Work out the finished part from the listing and answer in its coordinate system (mm). A direction names the side the tool comes from. Coordinates: 2 decimals unless noted, no trailing zeros. Loops run counter-clockwise (first coordinate to the right, second up) from the corner with the lowest first, then second, coordinate; pieces in that order, holes last. Notation, with made-up numbers: M 48,62 L 95,62 A27 ccw 95,97 Z; hole C 29,52 d9. An arc over 180 degrees is marked long. Write each question's results on one line, items separated by ' | '.
```python
from build123d import *

# Parameters (mm, degrees)
BOSS_EXTRUDE1_DEPTH = 1.8
SKETCH3_R           = 1.6
CUT_EXTRUDE1_DEPTH  = 31.775680334
SKETCH4_R           = 2.65
BOSS_EXTRUDE2_DEPTH = 4
SKETCH5_R           = 1.65
CUT_EXTRUDE2_DEPTH  = 31.98229333
SKETCH7_R           = 4.5
SKETCH7_R_2         = 3.5
BOSS_EXTRUDE4_DEPTH = 2.2
CHAMFER2_SIZE       = 1


with BuildPart() as part:
    # Sketch1 → Boss-Extrude1 (new body)
    with BuildSketch(Plane(origin=(0, 0, 0), x_dir=(1, 0, 0), z_dir=(0, 1, 0))):
        Polygon((0, 0.2), (23.05, 0.2), (23.05, 4.2), (29.05, 4.2), (29.05, 10), (0, 10), (0, 4.2), align=None)
    extrude(amount=BOSS_EXTRUDE1_DEPTH)

    # Sketch3 → Cut-Extrude1 (cut, through all)
    with BuildSketch(Plane.XZ):
        with Locations(Location((3.5, -3.689750901, 0), (0, 0, 270))):
            Circle(SKETCH3_R)
    extrude(amount=-CUT_EXTRUDE1_DEPTH, mode=Mode.SUBTRACT)

    # Sketch4 → Boss-Extrude2 (add)
    with BuildSketch(Plane.XZ):
        with Locations(Location((15, -4.689750901, 0), (0, 0, 270))):
            Circle(SKETCH4_R)
    extrude(amount=-BOSS_EXTRUDE2_DEPTH)

    # Sketch5 → Cut-Extrude2 (cut, through all)
    with BuildSketch(Plane(origin=(0, 4, 0), x_dir=(1, 0, 0), z_dir=(0, 1, 0))):
        with Locations(Location((15, 4.689750901, 0), (0, 0, 270))):
            Circle(SKETCH5_R)
    extrude(amount=-CUT_EXTRUDE2_DEPTH, mode=Mode.SUBTRACT)

    # Sketch7 → Boss-Extrude4 (add)
    with BuildSketch(Plane(origin=(0, 1.8, 0), x_dir=(1, 0, 0), z_dir=(0, 1, 0))):
        with Locations(Location((15, 4.689750901, 0), (0, 0, 90))):
            Circle(SKETCH7_R)
        with Locations(Location((15, 4.689750901, 0), (0, 0, 90))):
            Circle(SKETCH7_R_2, mode=Mode.SUBTRACT)
    extrude(amount=BOSS_EXTRUDE4_DEPTH)

    # Chamfer2
    chamfer2_edges = [part.edges().sort_by_distance(p)[0] for p in [
        (23.05, 1.8, -2.2),
        (29.05, 1.8, -7.1),
    ]]
    chamfer(chamfer2_edges, length=CHAMFER2_SIZE)


solid = part.part
```
1) Straight lines are drawn through the part: probe 1 along X at (y, z) = (3.75, -6.5); probe 2 along X at (y, z) = (3.65, -6.75); probe 3 along X at (y, z) = (3.7, -4.5). For each, find the intervals that lie inside material, in ascending order. Write a range as [from, to].
Check result:
probe 1: [10.88, 12], [13.06, 16.94], [18, 19.12] | probe 2: [11, 12.17], [13.33, 16.67], [17.83, 19] | probe 3: [10.5, 11.51], [12.36, 13.36], [16.64, 17.64], [18.49, 19.5]
2) Which of the six approach directions +Z, -Z, +X, -X, +Y, -Y give full straight-line access (tool end or side, diameter ignored) to faces 1 (the face through (22.56, 1.29, -2.17)), 2 (the face through (23.05, 0.4, -2.2)), 3 (the face through (11.2, 2.9, -7.1))?
Check result:
face 1: +Z, +X, +Y | face 2: +Z, +X, +Y, -Y | face 3: +Y
3) Find section B-B, the plane y = 1.5. Give the vertices of the cut face in (x, z), and give its area (3 significant figures).
Check result:
outline: M 0,-10 L 28.35,-10 L 28.35,-4.2 L 22.35,-4.2 L 22.35,-0.2 L 0,-0.2 Z; hole C 3.5,-3.69 d3.2; hole C 15,-4.69 d3.3 | area: 237 mm^2
4) Given pin 1 Ø2 at (x, y) = (10, 0.5) entering from +Z; pin 2 Ø1.4 at (x, y) = (24, 0.5) entering from +Z; pin 3 Ø1 at (y, z) = (1, -5.5) entering from -X; pin 4 Ø1 at (y, z) = (1.5, -5.5) entering from +X, each flat-ended and moving along its own axis, determine where each tip first touches the part or whether it passes through.
Check result:
pin 1: z = -0.2 | pin 2: z = -4.2 | pin 3: x = 0 | pin 4: x = 28.85
5) Find section C-C, the plane z = -2.5. Give the vertices of the cut face in (x, y).
Check result:
outline: M 0,0 L 2.43,0 L 2.43,1.8 L 0,1.8 Z; M 4.57,0 L 23.05,0 L 23.05,0.8 L 22.05,1.8 L 18.93,1.8 L 18.93,4 L 17.73,4 L 17.73,1.8 L 16.49,1.8 L 16.49,4 L 13.51,4 L 13.51,1.8 L 12.27,1.8 L 12.27,4 L 11.07,4 L 11.07,1.8 L 4.57,1.8 Z
6) Find section D-D, the plane x = 3.5. Give the vertices of the cut face in (y, z).
Check result:
outline: M 0,-10 L 1.8,-10 L 1.8,-5.29 L 0,-5.29 Z; M 0,-2.09 L 1.8,-2.09 L 1.8,-0.2 L 0,-0.2 Z
